Check sheet for the drawn part. Datum: minimum x, y, z corner. Units: mm. A direction names the side the tool comes from. Round coordinates to 2 decimals unless told otherwise and drop trailing zeros. Order: outer loops, then holes, each group sorted by start corner. A loop starts at its lowest first (then second) coordinate and runs counter-clockwise, first axis right, second up.
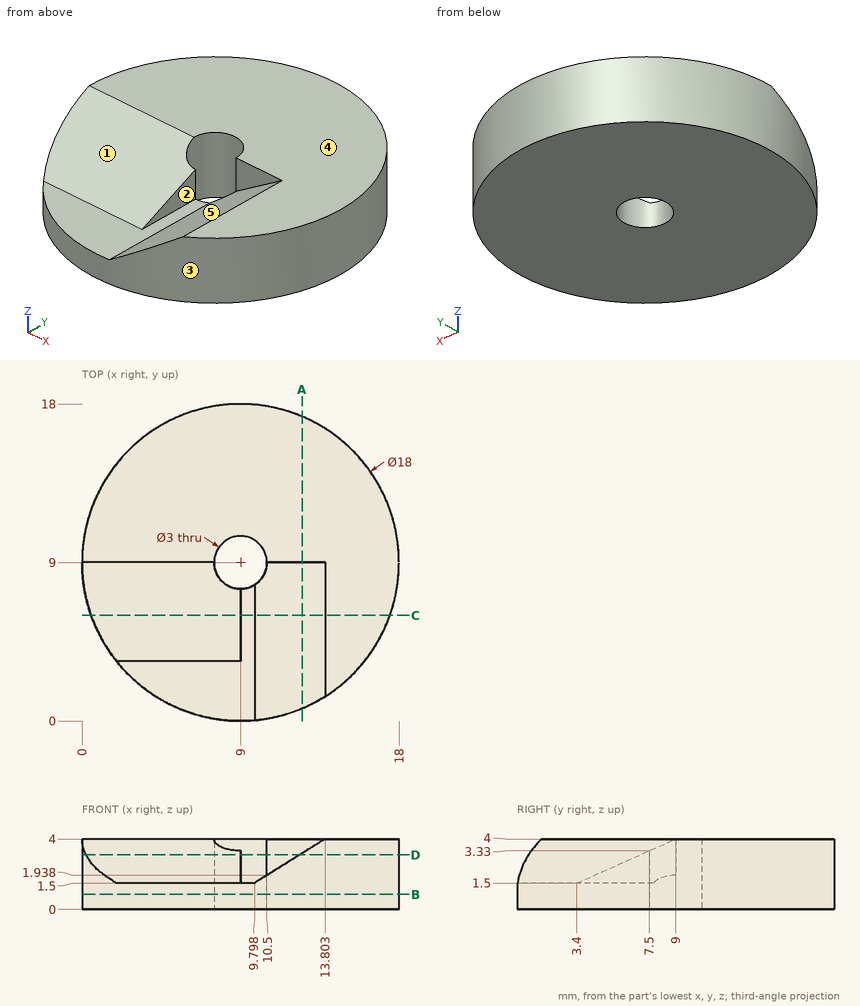
(1) Set-up check for the marked faces 4 and 5: record each of +Z, -Z, +X, -X, +Y, -Y from which the full face is reachable in a straight line by a thin tool's end or side.
Returned:
face 4: +Z, +X, -X, +Y, -Y
face 5: +Z, -Y
(2) Material ranges on line 1 (Y direction, x = 9, z = 1); line 2 (X direction, y = 7.75, z = 1.85) (1 decimal); line 3 (Y direction, x = 8.25, z = 0.9), recorded low to high.
Returned:
line 1: y = 0 to 7.5, 10.5 to 18
line 2: x = 0.1 to 8.2, 10.4 to 17.9
line 3: y = 0.03 to 7.7, 10.3 to 17.97
(3) Depth check by flat-ended pin: P1, Ø1.5, axis at x = 5, z = 2.5, coming from the -Y side; P2, Ø6, axis at x = 4.5, y = 3.5, coming from the +Z side (1 decimal); P3, Ø2, axis at y = 5, z = 2, coming from the +X side (1 decimal); P4, Ø2.5, axis at x = 9, y = 9, coming from the +Z side. Enter the tip coordinate at first touch or a pass-through.
Returned:
P1: stops at y = 3.96
P2: stops at z = 2.9
P3: stops at x = 17.5
P4: passes through
(4) Sectioned sample at C-C, the plane y = 6. Record the cut outline in (x, z) (1 decimal).
Returned:
outline: (0.5, 0) - (17.5, 0) - (17.5, 4) - (13.8, 4) - (9.8, 1.5) - (9, 1.5) - (9, 2.7) - (0.5, 2.7) - close
(5) Draft check along X on the marked faces 1, 2 and 3. Enter one of: released by +X, released by -X, zero draft, split by the parting line, or undercut.
Returned:
face 1: zero draft
face 2: undercut
face 3: split by the parting line
(6) Sectioned sample at A-A, the plane x = 12.5. Record the cut outline in (y, z).
Returned:
outline: (0.71, 0) - (17.29, 0) - (17.29, 4) - (9, 4) - (9, 3.19) - (0.71, 3.19) - close
(7) Sectioned sample at D-D, the plane z = 3.1. Record the cut outline in (x, y), and give its area (3 significant figures).
Returned:
outline: (0.23, 6.98) - (9, 6.98) - (9, 7.5) arc R1.5 cw (long way) to (10.5, 9) - (12.36, 9) - (12.36, 0.65) arc R9 ccw (long way) to start
area: 174 mm2
(8) Sectioned sample at B-B, the plane z = 0.85. Record the cut outline in (x, y).
Returned:
outline: circle Ø18 at (9, 9); hole circle Ø3 at (9, 9)
